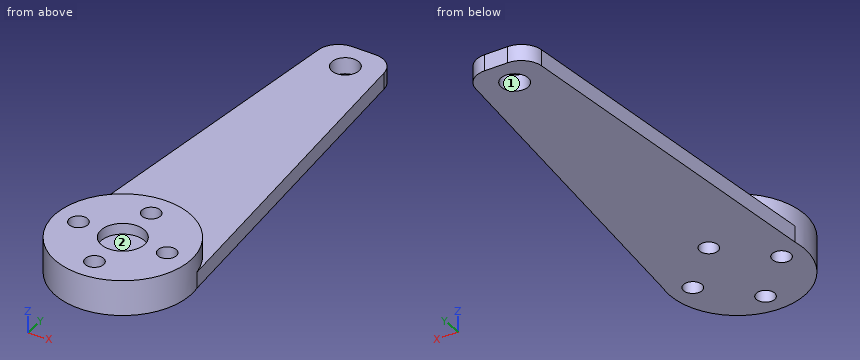
from build123d import *

# Parameters (mm, degrees)
ESQUISSE2_R                  = 12.5
BOSS_EXTRU_1_DEPTH           = 3.25
ESQUISSE3_R                  = 1.2
ENL_V_MAT_EXTRU_1_DEPTH      = 18.973939468
BOSS_EXTRU_2_DEPTH           = 3
ENL_V_MAT_EXTRU_2_DEPTH      = 72.455982989
ENL_V_MAT_EXTRU_2_DEPTH_BACK = 72.455982989
ESQUISSE10_R                 = 1.7
ESQUISSE17_R                 = 4
ENL_V_MAT_EXTRU_8_DEPTH      = 2
CONG_1_R                     = 4
ESQUISSE21_R                 = 2.5
ENL_V_MAT_EXTRU_9_DEPTH      = 72.455982989


with BuildPart() as part:
    # Esquisse2 → Boss.-Extru.1 (new, symmetric)
    with BuildSketch(Plane.XY):
        with Locations(Location((0, 0, 0), (0, 0, 180))):
            Circle(ESQUISSE2_R)
    extrude(amount=BOSS_EXTRU_1_DEPTH, both=True)

    # Esquisse3 → Enlèv. mat.-Extru.1 (cut, through all)
    with BuildSketch(Plane.XY):
        with Locations(Location((0, 8.25, 0), (0, 0, 180))):
            Circle(ESQUISSE3_R)
        with Locations(Location((-8.25, 0, 0), (0, 0, 180))):
            Circle(ESQUISSE3_R)
        with Locations(Location((0, -8.25, 0), (0, 0, 180))):
            Circle(ESQUISSE3_R)
        with Locations(Location((8.25, 0, 0), (0, 0, 180))):
            Circle(ESQUISSE3_R)
    extrude(amount=ENL_V_MAT_EXTRU_1_DEPTH, mode=Mode.SUBTRACT)

    # Esquisse20 → Boss.-Extru.2 (add)
    with BuildSketch(Plane(origin=(0, 0, -3.25), x_dir=(-1, 0, 0), z_dir=(0, 0, -1))):
        Polygon((-12.5, 0), (-5.772196938, 70.05324764), (5.772196938, 70.05324764), (12.5, 0), align=None)
    extrude(amount=-BOSS_EXTRU_2_DEPTH)

    # Esquisse10 → Enlèv. mat.-Extru.2 (cut, two sides: drawn at the far end of the back side and taken through both)
    with BuildSketch(Plane(origin=(0, 0, -3.25), x_dir=(-1, 0, 0), z_dir=(0, 0, -1)).offset(-ENL_V_MAT_EXTRU_2_DEPTH_BACK)):
        with Locations((-8.25, 0)):
            Circle(ESQUISSE10_R)
        with Locations((0, 8.25)):
            Circle(ESQUISSE10_R)
        with Locations((8.25, 0)):
            Circle(ESQUISSE10_R)
        with Locations((0, -8.25)):
            Circle(ESQUISSE10_R)
    extrude(amount=ENL_V_MAT_EXTRU_2_DEPTH + ENL_V_MAT_EXTRU_2_DEPTH_BACK, mode=Mode.SUBTRACT)

    # Esquisse17 → Enlèv. mat.-Extru.8 (cut)
    with BuildSketch(Plane.XY.offset(3.25)):
        Circle(ESQUISSE17_R)
    extrude(amount=-ENL_V_MAT_EXTRU_8_DEPTH, mode=Mode.SUBTRACT)

    # Congé1
    cong_1_edges = [part.edges().sort_by_distance(p)[0] for p in [
        (-5.772196938, 70.05324764, -1.75),
        (5.772196938, 70.05324764, -1.75),
    ]]
    fillet(cong_1_edges, radius=CONG_1_R)

    # Esquisse21 → Enlèv. mat.-Extru.9 (cut, through all)
    with BuildSketch(Plane(origin=(0, 0, -3.25), x_dir=(-1, 0, 0), z_dir=(0, 0, -1))):
        with Locations((0, 64.696529063)):
            Circle(ESQUISSE21_R)
    extrude(amount=-ENL_V_MAT_EXTRU_9_DEPTH, mode=Mode.SUBTRACT)


solid = part.part
Part model, mm, in its own coordinate system. Face numbers are marked on the shaded views. A direction names the side the tool comes from. Give positions to 0.01 mm unless a question says otherwise; leave off trailing zeros. Loops run counter-clockwise (first coordinate to the right, second up) from the corner with the lowest first, then second, coordinate; pieces in that order, holes last. Notation, with made-up numbers: M 51,50.5 L 88,50.5 A20 cw 88,80.5 Z; hole C 8,-6 d7. An arc over 180 degrees is marked long. Put each result on its own line as item: value. Start each with the question number.
1) Saw through at B-B (y = 0). List the corners of the cut face in (x, z).
2) 3-axis set-ups, long thin cutter, end or side, ignore diameter. For the marked faces 1 and 2: which of +Z, -Z, +X, -X, +Y, -Y reach the whole face in a straight line?
3) Saw through at D-D (x = 8.5). List the corners of the cut face in (y, z), then the cut area to 3 significant figures.
4) Probe probe 1 along Y at (x, z) = (0, -0.75); probe 2 along Y at (x, z) = (0, 2.8); probe 3 along Z at (x, y) = (-1.25, 21.5). List the from-to ranges inside material, lowest first.
5) Flat gauge pins, fed straight in: pin 1 (5.5 mm diameter, centred on x = 8.25, y = 0, fed in from -Z); pin 2 (4 mm diameter, centred on x = 0, y = 64.7, fed in from -Z); pin 3 (8 mm diameter, centred on x = -5, y = 46.5, fed in from +Z); pin 4 (3 mm diameter, centred on x = 5.5, z = -1.5, fed in from +Y). Where does each tip first touch, or does it go through?
6) Saw through at A-A (x = 0). List the corners of the cut face in (y, z).
7) Saw through at C-C (z = 2). List the corners of the cut face in (x, y).
Numbers:
1. outline: M -12.5,-3.25 L -9.95,-3.25 L -9.95,3.25 L -12.5,3.25 Z; M -6.55,-3.25 L 6.55,-3.25 L 6.55,3.25 L 4,3.25 L 4,1.25 L -4,1.25 L -4,3.25 L -6.55,3.25 Z; M 9.95,-3.25 L 12.5,-3.25 L 12.5,3.25 L 9.95,3.25 Z
2. face 1: +Z, -Z
2. face 2: +Z
3. outline: M -9.17,-3.25 L -1.68,-3.25 L -1.68,3.25 L -9.17,3.25 Z; M 1.68,-3.25 L 41.65,-3.25 L 41.65,-0.25 L 9.17,-0.25 L 9.17,3.25 L 1.68,3.25 Z
3. area: 195 mm^2
4. probe 1: -12.5 to -9.95, -6.55 to 6.55, 9.95 to 62.2, 67.2 to 70.05
4. probe 2: -12.5 to -9.95, -6.55 to -4, 4 to 6.55, 9.95 to 12.5
4. probe 3: -3.25 to -0.25
5. pin 1: z = -3.25
5. pin 2: through
5. pin 3: z = -0.25
5. pin 4: y = 69.59
6. outline: M -12.5,-3.25 L -9.95,-3.25 L -9.95,3.25 L -12.5,3.25 Z; M -6.55,-3.25 L 6.55,-3.25 L 6.55,3.25 L 4,3.25 L 4,1.25 L -4,1.25 L -4,3.25 L -6.55,3.25 Z; M 9.95,-3.25 L 62.2,-3.25 L 62.2,-0.25 L 12.5,-0.25 L 12.5,3.25 L 9.95,3.25 Z; M 67.2,-3.25 L 70.05,-3.25 L 70.05,-0.25 L 67.2,-0.25 Z
7. outline: C 0,0 d25; hole C -8.25,0 d3.4; hole C 0,0 d8; hole C 0,-8.25 d3.4; hole C 0,8.25 d3.4; hole C 8.25,0 d3.4
